Check sheet for the drawn part. Datum: minimum x, y, z corner. Units: mm. Round coordinates to 2 decimals unless told otherwise and drop trailing zeros. Write each loop counter-clockwise with the first axis right and the second up, starting at its lowest first coordinate (ties: lowest second). Pieces come first, ordered by that corner, then holes. Notation, with made-up numbers: (46, 31) - (98, 31) arc R16 ccw to (98, 50) - close; hole circle Ø10 at (-14.75, 77.25). An arc over 180 degrees is marked (long way). Return JSON: item names as keys, results as strings. Group by question number.
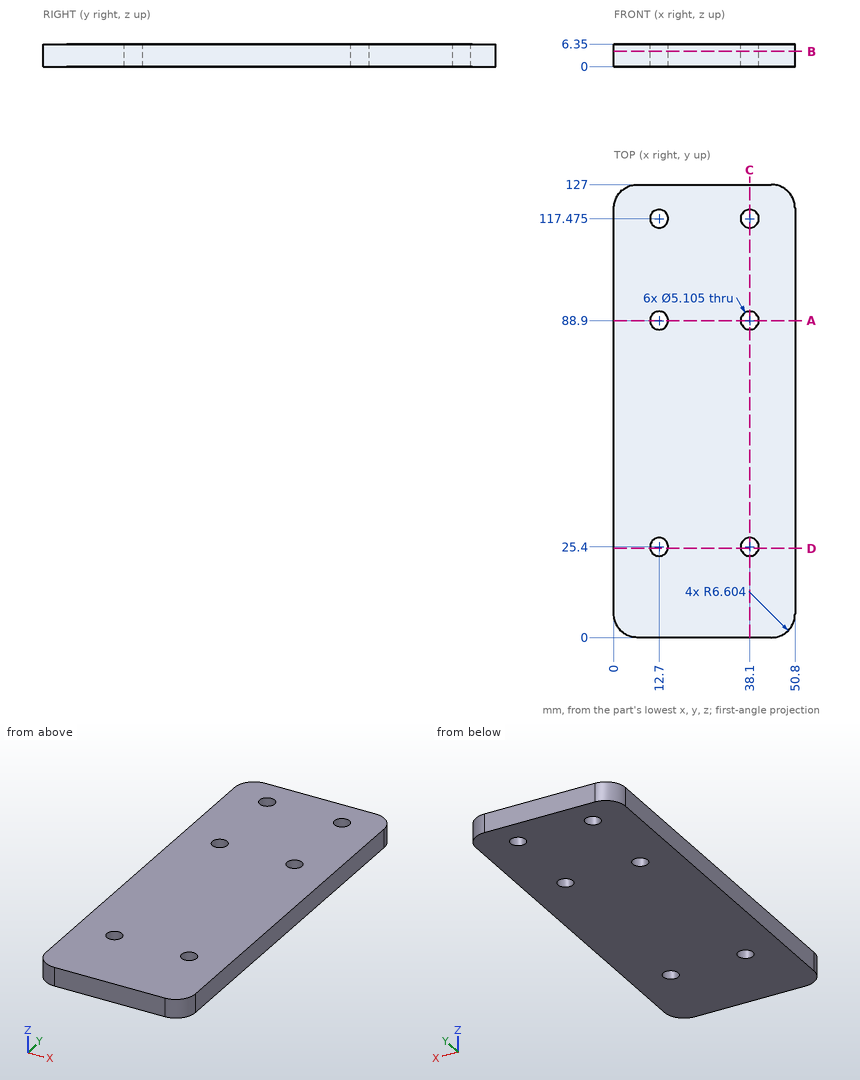
1. Section check C-C (x = 38.1). Enter the section's corners in (y, z), and give its area (3 significant figures).
2. Section check D-D (y = 25). Enter the section's corners in (x, z).
3. Section check B-B (z = 4.25). Enter the section's corners in (x, y) (1 decimal).
4. Depth check by flat-ended pin: pin 1 Ø8 at (x, y) = (12.7, 88.9) entering from +Z; pin 2 Ø4 at (x, y) = (38.1, 88.9) entering from -Z. Enter the tip coordinate at first touch or a pass-through.
5. Material ranges on line 1 along Y through (x, z) = (38.1, 4); line 2 along X through (y, z) = (25.4, 1.5); line 3 along Y through (x, z) = (13, 2.5) (1 decimal), recorded low to high.
6. Section check A-A (y = 88.9). Enter the section's corners in (x, z), and give its area (3 significant figures).
Result sheet:
{
 "1": {"outline": "(0, 0) - (22.85, 0) - (22.85, 6.35) - (0, 6.35) - close; (27.95, 0) - (86.35, 0) - (86.35, 6.35) - (27.95, 6.35) - close; (91.45, 0) - (114.92, 0) - (114.92, 6.35) - (91.45, 6.35) - close; (120.03, 0) - (127, 0) - (127, 6.35) - (120.03, 6.35) - close", "area": "709 mm²"},
 "2": {"outline": "(0, 0) - (10.18, 0) - (10.18, 6.35) - (0, 6.35) - close; (15.22, 0) - (35.58, 0) - (35.58, 6.35) - (15.22, 6.35) - close; (40.62, 0) - (50.8, 0) - (50.8, 6.35) - (40.62, 6.35) - close"},
 "3": {"outline": "(0, 6.6) arc R6.6 ccw to (6.6, 0) - (44.2, 0) arc R6.6 ccw to (50.8, 6.6) - (50.8, 120.4) arc R6.6 ccw to (44.2, 127) - (6.6, 127) arc R6.6 ccw to (0, 120.4) - close; hole circle Ø5.1 at (12.7, 25.4); hole circle Ø5.1 at (12.7, 88.9); hole circle Ø5.1 at (12.7, 117.5); hole circle Ø5.1 at (38.1, 25.4); hole circle Ø5.1 at (38.1, 88.9); hole circle Ø5.1 at (38.1, 117.5)"},
 "4": {"pin 1": "stops at z = 6.35", "pin 2": "passes through"},
 "5": {"line 1": "y = 0 to 22.85, 27.95 to 86.35, 91.45 to 114.92, 120.03 to 127", "line 2": "x = 0 to 10.15, 15.25 to 35.55, 40.65 to 50.8", "line 3": "y = 0 to 22.9, 27.9 to 86.4, 91.4 to 114.9, 120 to 127"},
 "6": {"outline": "(0, 0) - (10.15, 0) - (10.15, 6.35) - (0, 6.35) - close; (15.25, 0) - (35.55, 0) - (35.55, 6.35) - (15.25, 6.35) - close; (40.65, 0) - (50.8, 0) - (50.8, 6.35) - (40.65, 6.35) - close", "area": "258 mm²"}
}
